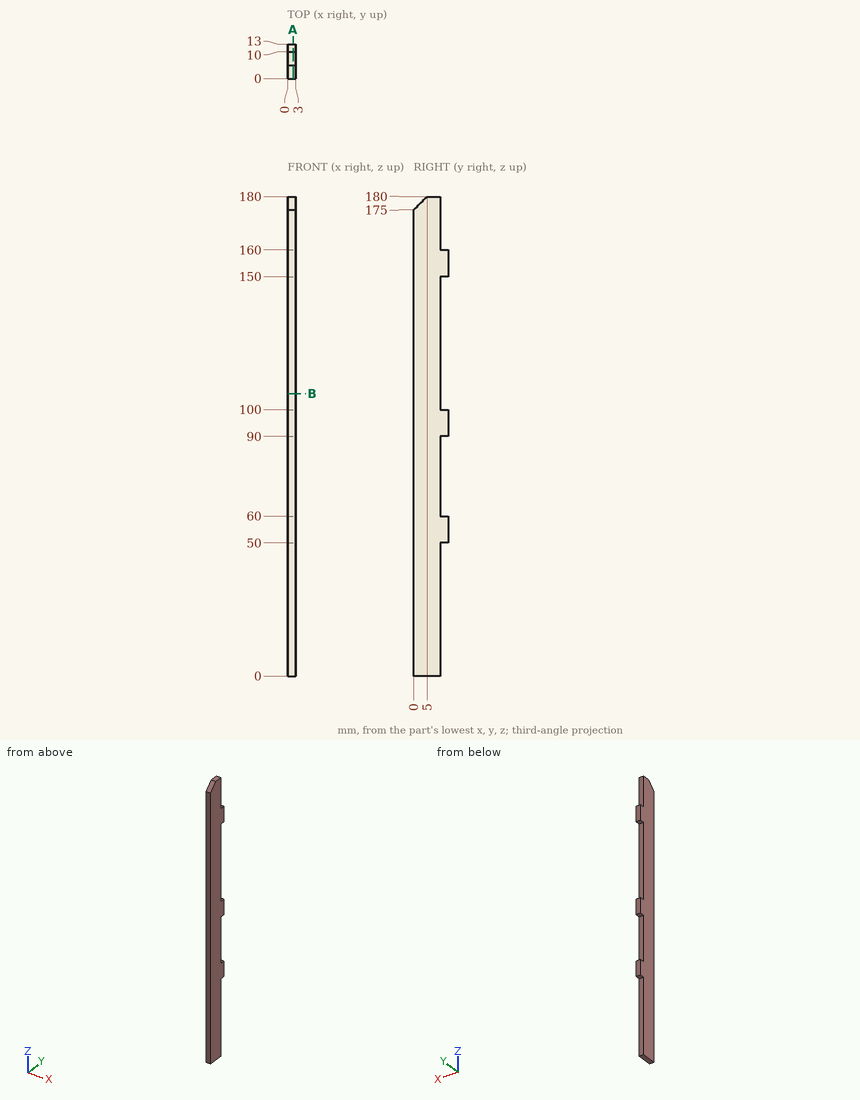
Print and shaded views of the part. All mm, measured from the part's lowest x, y and z. Give positions to 0.01 mm unless a question says otherwise; leave off trailing zeros. Loops run counter-clockwise (first coordinate to the right, second up) from the corner with the lowest first, then second, coordinate; pieces in that order, holes last.
1) Saw through at B-B (z = 106). Write the cut outline in (x, y), plus the area to 3 significant figures.
2) Saw through at A-A (x = 2). Write the cut outline in (y, z).
3) Flat gauge pins, fed straight in: pin 1 Ø0.9 at (x, y) = (2, 11.5) entering from -Z; pin 2 Ø1.5 at (x, y) = (1.5, 11.5) entering from +Z; pin 3 Ø0.9 at (x, z) = (1.5, 119) entering from +Y. Where does each tip first touch, or does it go through?
4) Wall check: line 1 (Z direction, x = 1.1, y = 11.5); line 2 (Y direction, x = 2.65, z = 165.5); line 3 (Z direction, x = 1.1, y = 2). Give the ranges that are in metal, low to high.
Answer block:
1. outline: (0, 0) - (3, 0) - (3, 10) - (0, 10) - close
1. area: 30.0 mm2
2. outline: (0, 0) - (10, 0) - (10, 50) - (13, 50) - (13, 60) - (10, 60) - (10, 90) - (13, 90) - (13, 100) - (10, 100) - (10, 150) - (13, 150) - (13, 160) - (10, 160) - (10, 180) - (5, 180) - (0, 175) - close
3. pin 1: stops at z = 50
3. pin 2: stops at z = 160
3. pin 3: stops at y = 10
4. line 1: z = 50 to 60, 90 to 100, 150 to 160
4. line 2: y = 0 to 10
4. line 3: z = 0 to 177
